Input: part model. Units: mm. Frame: model coordinates. Face numbers are marked on the shaded views. A direction names the side the tool comes from. Coordinates: 2 decimals unless noted, no trailing zeros. Loops run counter-clockwise (first coordinate to the right, second up) from the corner with the lowest first, then second, coordinate; pieces in that order, holes last. Notation, with made-up numbers: (71, 12) - (90, 12) arc R21 cw to (90, 51) - close; hole circle Ø7 at (-32, 11.25). An arc over 180 degrees is marked (long way). Use a Markdown table: item, result. Add a question column.
1. Contact query for flat-ended pins moving along their axis: P1, Ø8, axis at x = -1, y = -6, coming from the -Z side; P2, Ø2, axis at y = -3.5, z = 21.5, coming from the -X side; P3, Ø6, axis at x = -1.5, z = 22.5, coming from the -Y side. Output: stop coordinate, or through.
2. Section query C-C on x = -1. Return the cut outline in (y, z), then the cut area to 3 significant figures.
3. Section query A-A on y = 0. Return the cut outline in (x, z), then the cut area to 3 significant figures.
4. Ray query, L1, parallel to Y at x = 0, z = 20.75; L2, parallel to Y at x = 0, z = 7.25; L3, parallel to Z at x = 2, y = 0.75. Return the intervals inside material, ascending. Write a range as [from, to].
5. Draft query along X for the marked faces 1, 2, 3 and 4. Return one class per face: released by +X, released by -X, zero draft, split by the parting line, or undercut.
6. Section query B-B on z = 3.5. Return the cut outline in (x, y) (1 decimal).
7. Section query D-D on y = 5.5. Return the cut outline in (x, z).
8. Access query for the marked faces 5, 6 and 7. Directions: +Z, -Z, +X, -X, +Y, -Y. A direction counts if a zero-diameter tool reaches every point of the face in a straight line with its end or side. Return the directions, or none.
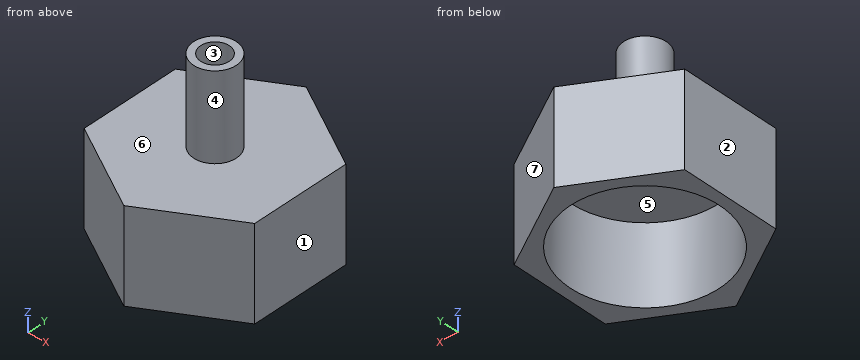
```python
from build123d import *

# Parameters (mm, degrees)
HEX_NUT_DEPTH     = 13
SKETCH2_R         = 10.4775
THREAD_BORE_DEPTH = 11
BARB_START        = 13
SKETCH3_R         = 3
BARB_DEPTH        = 12
SKETCH4_R         = 2
BORE_DEPTH        = 32


with BuildPart() as part:
    # Sketch1 → Hex_Nut (new body)
    with BuildSketch(Plane.XY):
        Polygon((12, 6.92820323), (0, 13.856406461), (-12, 6.92820323), (-12, -6.92820323), (0, -13.856406461), (12, -6.92820323), align=None)
    extrude(amount=HEX_NUT_DEPTH)

    # Sketch2 → Thread_Bore (cut)
    with BuildSketch(Plane.XY):
        Circle(SKETCH2_R)
    extrude(amount=THREAD_BORE_DEPTH, mode=Mode.SUBTRACT)

    # Sketch3 → Barb (add)
    with BuildSketch(Plane.XY.offset(BARB_START)):
        Circle(SKETCH3_R)
    extrude(amount=BARB_DEPTH)

    # Sketch4 → Bore (cut, through all)
    with BuildSketch(Plane.XY):
        Circle(SKETCH4_R)
    extrude(amount=BORE_DEPTH, mode=Mode.SUBTRACT)


solid = part.part
```
Resolved:
| question | item | result |
|---|---|---|
| 1 | P1 | z = 11 |
| 1 | P2 | x = -1.66 |
| 1 | P3 | y = -3 |
| 2 | outline | (-13.28, 0) - (-10.43, 0) - (-10.43, 11) - (-1.73, 11) - (-1.73, 25) - (-2.83, 25) - (-2.83, 13) - (-13.28, 13) - close; (1.73, 11) - (10.43, 11) - (10.43, 0) - (13.28, 0) - (13.28, 13) - (2.83, 13) - (2.83, 25) - (1.73, 25) - close |
| 2 | area | 135 mm² |
| 3 | outline | (-12, 0) - (-10.48, 0) - (-10.48, 11) - (-2, 11) - (-2, 25) - (-3, 25) - (-3, 13) - (-12, 13) - close; (2, 11) - (10.48, 11) - (10.48, 0) - (12, 0) - (12, 13) - (3, 13) - (3, 25) - (2, 25) - close |
| 3 | area | 97.5 mm² |
| 4 | L1 | [-3, -2], [2, 3] |
| 4 | L2 | [-13.86, -10.48], [10.48, 13.86] |
| 4 | L3 | [11, 25] |
| 5 | face 1 | released by +X |
| 5 | face 2 | released by -X |
| 5 | face 3 | undercut |
| 5 | face 4 | split by the parting line |
| 6 | outline | (-12, -6.9) - (0, -13.9) - (12, -6.9) - (12, 6.9) - (0, 13.9) - (-12, 6.9) - close; hole circle Ø21 at (0, 0) |
| 7 | outline | (-12, 0) - (-8.92, 0) - (-8.92, 11) - (8.92, 11) - (8.92, 0) - (12, 0) - (12, 13) - (-12, 13) - close |
| 8 | face 5 | -Z |
| 8 | face 6 | +Z |
| 8 | face 7 | +Z, -Z, +X, +Y |
